```python
from build123d import *

# Parameters (mm, degrees)
F0_R     = 7.5
F0_R_2   = 25
F0_R_3   = 13
F1_DEPTH = 25


with BuildPart() as f1:
    # F0 (on Front) → F1 (new body)
    with BuildSketch(Plane.XZ):
        with BuildLine():
            ThreePointArc((7.980277, 56.438596), (0, 49), (-7.980277, 56.438596))
            ThreePointArc((-7.980277, 56.438596), (-57, 0), (-7.980277, -56.438596))
            ThreePointArc((-7.980277, -56.438596), (0, -49), (7.980277, -56.438596))
            ThreePointArc((7.980277, -56.438596), (57, 0), (7.980277, 56.438596))
        make_face()
        with Locations((-28.991378, -28.991378)):
            Circle(F0_R, mode=Mode.SUBTRACT)
        with Locations((28.991378, -28.991378)):
            Circle(F0_R, mode=Mode.SUBTRACT)
        Circle(F0_R_2, mode=Mode.SUBTRACT)
        with Locations((-28.991378, 28.991378)):
            Circle(F0_R, mode=Mode.SUBTRACT)
        with Locations((28.991378, 28.991378)):
            Circle(F0_R, mode=Mode.SUBTRACT)
        Circle(F0_R_2)
        Circle(F0_R_3, mode=Mode.SUBTRACT)
    extrude(amount=F1_DEPTH)


solid = f1.part
```
The listing builds one solid part. Answer for the finished solid, in the listing's coordinates (mm). Give positions to 0.01 mm unless a question says otherwise; leave off trailing zeros. Order: outer loops, then holes, each group sorted by start corner. A loop starts at its lowest first (then second) coordinate and runs counter-clockwise, first axis right, second up. Notation, with made-up numbers: (68.25, 34) - (112.25, 34) arc R21 ccw to (112.25, 43) - close; hole circle Ø9 at (15.5, 21.25). An arc over 180 degrees is marked (long way). Answer in a Markdown table with one row per item. Add a question column.
Q1. The part is cut by section A-A (x = 0). Determine the outline of the cut face in (y, z).
Q2. Find the intervals of material crossed by line 1 along X through (y, z) = (-4, -24.5); line 2 along Z through (x, y) = (0, -1.5); line 3 along X through (y, z) = (-10.25, 30), in increasing order. Write a range as [from, to].
Q3. The part is cut by section C-C (y = -15). Determine the outline of the cut face in (x, z), then the cut area to 3 significant figures.
Q4. For a pull along X with two mould halves and no side action, classify faces 1 (the cylindrical face through (-56.99, -12.32, 1.14)), 2 (the cylindrical face through (-10.316, -12.325, -7.91)), 3 (the flat face through (-0.8, -25, 13.3)) as released by +X, released by -X, zero draft, split by the parting line, or undercut.
Q5. Given P1, Ø4, axis at x = 0.5, y = -22.5, coming from the +Z side; P2, Ø10, axis at x = 22, y = -11, coming from the +Z side; P3, Ø10, axis at y = -6.5, z = -43.5, coming from the -X side, each flat-ended and moving along its own axis, determine where each tip first touches the part or whether it passes through.
Q6. The part is cut by section D-D (z = -25). Determine the outline of the cut face in (x, y) (3 decimals), then the cut area to 3 significant figures.
Q7. The part is cut by section B-B (z = 0). Determine the outline of the cut face in (x, y).
Determined:
| question | item | result |
|---|---|---|
| 1 | outline | (-25, -49) - (0, -49) - (0, -13) - (-25, -13) - close; (-25, 13) - (0, 13) - (0, 49) - (-25, 49) - close |
| 2 | line 1 | x = [-51.47, -35], [-22.98, 22.98], [35, 51.47] |
| 2 | line 2 | z = [-49, -13], [13, 49] |
| 2 | line 3 | x = [-48.47, -36.42], [-21.56, 21.56], [36.42, 48.47] |
| 3 | outline | (-7.98, -56.44) arc R8 cw to (7.98, -56.44) arc R57 ccw to (7.98, 56.44) arc R8 cw to (-7.98, 56.44) arc R57 ccw to start; hole circle Ø15 at (-28.99, -28.99); hole circle Ø15 at (-28.99, 28.99); hole circle Ø26 at (0, 0); hole circle Ø15 at (28.99, -28.99); hole circle Ø15 at (28.99, 28.99) |
| 3 | area | 8,770 mm² |
| 4 | face 1 | released by -X |
| 4 | face 2 | undercut |
| 4 | face 3 | zero draft |
| 5 | P1 | stops at z = 49.4 |
| 5 | P2 | stops at z = 54.41 |
| 5 | P3 | stops at x = -42.03 |
| 6 | outline | (-51.225, -25) - (-35.341, -25) - (-35.341, 0) - (-51.225, 0) - close; (-22.642, -25) - (22.642, -25) - (22.642, 0) - (-22.642, 0) - close; (35.341, -25) - (51.225, -25) - (51.225, 0) - (35.341, 0) - close |
| 6 | area | 1,930 mm² |
| 7 | outline | (-57, -25) - (-13, -25) - (-13, 0) - (-57, 0) - close; (13, -25) - (57, -25) - (57, 0) - (13, 0) - close |
